Can you work these out from the model? Positions are in its coordinate system, mm. Face numbers are marked on the shaded views. A direction names the side the tool comes from. Coordinates: 2 decimals unless noted, no trailing zeros. Loops run counter-clockwise (first coordinate to the right, second up) from the corner with the lowest first, then second, coordinate; pieces in that order, holes last.
```python
from build123d import *

# Parameters (mm, degrees)
SKETCH1_W           = 23.127
SKETCH1_H           = 16.5
SKETCH1_W_2         = 13.127
SKETCH1_H_2         = 5.5
SKETCH1_W_3         = 2.55
SKETCH1_H_3         = 6
BOSS_EXTRUDE1_DEPTH = 24.5
SKETCH2_W           = 2.55
SKETCH2_H           = 6
CUT_EXTRUDE1_DEPTH  = 2
SKETCH3_W           = 13.127
SKETCH3_H           = 5
CUT_EXTRUDE2_DEPTH  = 15


with BuildPart() as part:
    # Sketch1 → Boss-Extrude1 (new body)
    # profile 1 of 2: a face of its own
    with BuildSketch(Plane(origin=(0, 0, 0), x_dir=(1, 0, 0), z_dir=(0, 1, 0))):
        with Locations((-1.462471661, -2.897695951)):
            Rectangle(SKETCH1_W, SKETCH1_H)
        with Locations((-1.462471661, -3.397695951)):
            Rectangle(SKETCH1_W_2, SKETCH1_H_2, mode=Mode.SUBTRACT)
    # profile 2 of 2: a face of its own
    with BuildSketch(Plane(origin=(0, 0, 0), x_dir=(1, 0, 0), z_dir=(0, 1, 0))):
        with Locations((-1.462471661, 2.352304049)):
            Rectangle(SKETCH1_W_3, SKETCH1_H_3)
    extrude(amount=BOSS_EXTRUDE1_DEPTH)

    # Sketch2 → Cut-Extrude1 (cut)
    with BuildSketch(Plane.XZ):
        with Locations((-1.462471661, -2.352304049)):
            Rectangle(SKETCH2_W, SKETCH2_H)
    extrude(amount=-CUT_EXTRUDE1_DEPTH, mode=Mode.SUBTRACT)

    # Sketch3 → Cut-Extrude2 (cut)
    with BuildSketch(Plane(origin=(0, 24.5, 0), x_dir=(1, 0, 0), z_dir=(0, 1, 0))):
        with Locations((-1.462471661, -8.647695951)):
            Rectangle(SKETCH3_W, SKETCH3_H)
    extrude(amount=-CUT_EXTRUDE2_DEPTH, mode=Mode.SUBTRACT)


solid = part.part
```
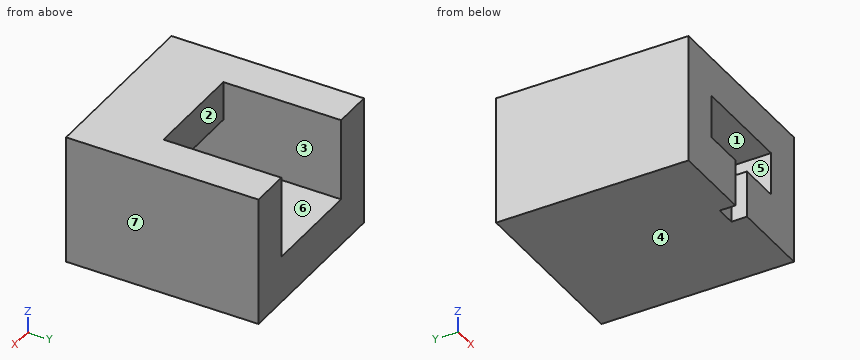
Item 1: We'd pull the mould along X, two halves only. Please class the marked faces 4, 5, 6 and 7: +X half, -X half, draft (parallel to the pull), parting line (faces both ways), or undercut.
Results are:
face 4: draft
face 5: undercut
face 6: undercut
face 7: +X half
Item 2: On a 3-axis mill with a long thin cutter (end or side, diameter ignored), from which of +Z, -Z, +X, -X, +Y, -Y can I reach the whole of each face in a straight line? I mean the marked faces 1, 2 and 3. Say none if no direction works.
Results are:
face 1: +Y, -Y
face 2: +Z, +Y
face 3: +Y
Item 3: Suppose I cut it at D-D, the plane z = 7.25. Please give me the cut outline in (x, y).
Results are:
outline: (-13.03, 0) - (10.1, 0) - (10.1, 24.5) - (5.1, 24.5) - (5.1, 9.5) - (-8.03, 9.5) - (-8.03, 24.5) - (-13.03, 24.5) - close
Item 4: Suppose I cut it at B-B, the plane z = 5.25. Please give me the cut outline in (x, y), plus the area to 3 significant figures.
Results are:
outline: (-13.03, 0) - (-8.03, 0) - (-8.03, 24.5) - (-13.03, 24.5) - close; (5.1, 0) - (10.1, 0) - (10.1, 24.5) - (5.1, 24.5) - close
area: 245 mm2
Item 5: Suppose I cut it at C-C, the plane y = 20.75. Please give me the cut outline in (x, z).
Results are:
outline: (-13.03, -5.35) - (10.1, -5.35) - (10.1, 11.15) - (5.1, 11.15) - (5.1, 0.65) - (-8.03, 0.65) - (-8.03, 11.15) - (-13.03, 11.15) - close
Item 6: I need wall thicknesses on line 1 along X through (y, z) = (12, 3.75); line 2 along Z through (x, y) = (-5.5, 5.75); line 3 along X through (y, z) = (1.75, -2.75). Which ranges of each line are inside material? Lowest first, please.
Results are:
line 1: x = -13.03 to -8.03, 5.1 to 10.1
line 2: z = -5.35 to 0.65, 6.15 to 11.15
line 3: x = -13.03 to -2.74, -0.19 to 10.1
Item 7: Suppose I cut it at A-A, the plane x = 3.75. Please give me the cut outline in (y, z), plus the area to 4 significant figures.
Results are:
outline: (0, -5.35) - (24.5, -5.35) - (24.5, 0.65) - (0, 0.65) - close; (0, 6.15) - (9.5, 6.15) - (9.5, 11.15) - (0, 11.15) - close
area: 194.5 mm2
Item 8: I'm going to push flat-ended pins straight in: P1, Ø4, axis at x = -3.5, y = 18, coming from the +Z side; P2, Ø2.5, axis at x = 1.5, z = 9, coming from the +Y side. Where does each tip first touch, or does it pass through?
Results are:
P1: stops at z = 0.65
P2: stops at y = 9.5
